Source: CAD feature listing. Evaluate the final solid. Frame: model axes, mm. A direction names the side the tool comes from. Round coordinates to 2 decimals unless told otherwise and drop trailing zeros. Write each loop counter-clockwise with the first axis right and the second up, starting at its lowest first coordinate (ties: lowest second). Pieces come first, ordered by that corner, then holes. Notation, with made-up numbers: M 81.5,79 L 87.5,79 A6 ccw 87.5,84 Z; hole C 69.25,19 d7. An arc over 180 degrees is marked long. Answer in a Markdown table with one row per item. Add a question column.
Item 1: Cut plane D-D on z = 0. Give the number of separate pieces and of enclosed holes in the cut face, and give its area (3 significant figures).
Item 2: Cut plane C-C on y = -10.75. Return loops of the section in (x, z), and give its area (3 significant figures).
Item 3: Cut plane B-B on z = 21.5. Return loops of the section in (x, y), and give its area (3 significant figures).
Item 4: Material intervals for probe 1 along X at (y, z) = (-14.45, 0); probe 2 along Y at (x, z) = (-3, -6.5); probe 3 along Z at (x, y) = (0, -0.9), sorted ascending.
Item 5: Contact query for flat-ended pins moving along their axis: pin 1 (2.5 mm diameter, centred on x = -30, z = 0, fed in from +Y); pin 2 (25 mm diameter, centred on x = -4, z = 11, fed in from +Y); pin 3 (1 mm diameter, centred on x = -28, y = -4, fed in from -Z). Output: stop coordinate, or through.
Item 6: Cut plane A-A on x = 30. Return loops of the section in (y, z).
Item 7: Mould query, pull axis Z, two halves, no side actions, for faces 3 (the face through (0, -1, -2)), 4 (the face through (-50, -14, 9)), 5 (the face through (-35, -7, 28.5)). Classes: released by +Z, released by -Z, zero draft, split by the parting line, or undercut.
Item 8: Set-up query: faces 1 (the face through (-1, 0, 5)), 2 (the face through (42, -7, 28.5)). Return all of +Z, -Z, +X, -X, +Y, -Y with unobstructed straight access to the full face (end or side cutting, diameter ignored); none if empty.
from build123d import *

# Parameters (mm, degrees)
F0_W     = 100
F0_H     = 50
F0_R     = 2
F0_R_2   = 2.212138
F1_DEPTH = 15
F2_W     = 12
F2_H     = 48.5
F3_DEPTH = 100.001
F4_W     = 55
F4_H     = 12
F5_DEPTH = 25


with BuildPart() as f1:
    # F0 (on Front) → F1 (new body)
    with BuildSketch(Plane.XZ):
        with Locations((0, 5)):
            Rectangle(F0_W, F0_H)
        with Locations((-30, 0)):
            Circle(F0_R, mode=Mode.SUBTRACT)
        Circle(F0_R, mode=Mode.SUBTRACT)
        with Locations((30, 0)):
            Circle(F0_R, mode=Mode.SUBTRACT)
        with Locations((20, 25)):
            Circle(F0_R_2, mode=Mode.SUBTRACT)
    extrude(amount=F1_DEPTH)

    # F2 (on face) → F3 (cut, through all)
    with BuildSketch(Plane(origin=(-50, 0, 0), x_dir=(0, -1, 0), z_dir=(-1, 0, 0))):
        with Locations((7.5, 4.25)):
            Rectangle(F2_W, F2_H)
    extrude(amount=-F3_DEPTH, mode=Mode.SUBTRACT)

    # F4 (on face) → F5 (cut)
    with BuildSketch(Plane.XY.offset(30)):
        with Locations((7.5, -7.5)):
            Rectangle(F4_W, F4_H)
    extrude(amount=-F5_DEPTH, mode=Mode.SUBTRACT)


solid = f1.part
Results below:
| question | item | result |
|---|---|---|
| 1 | separate pieces | 8 |
| 1 | enclosed holes | 0 |
| 1 | area | 264 mm2 |
| 2 | outline | M -50,28.5 L -20,28.5 L -20,30 L -50,30 Z; M 35,28.5 L 50,28.5 L 50,30 L 35,30 Z |
| 2 | area | 67.5 mm2 |
| 3 | outline | M -50,-15 L 50,-15 L 50,-13.5 L -50,-13.5 Z; M -50,-1.5 L 50,-1.5 L 50,0 L -50,0 Z |
| 3 | area | 300 mm2 |
| 4 | probe 1 | -50 to -32, -28 to -2, 2 to 28, 32 to 50 |
| 4 | probe 2 | -15 to -13.5, -1.5 to 0 |
| 4 | probe 3 | -20 to -2, 2 to 30 |
| 5 | pin 1 | through |
| 5 | pin 2 | y = 0 |
| 5 | pin 3 | z = 28.5 |
| 6 | outline | M -15,-20 L -13.5,-20 L -13.5,-2 L -15,-2 Z; M -15,2 L -13.5,2 L -13.5,30 L -15,30 Z; M -1.5,-20 L 0,-20 L 0,-2 L -1.5,-2 Z; M -1.5,2 L 0,2 L 0,30 L -1.5,30 Z |
| 7 | face 3 | undercut |
| 7 | face 4 | zero draft |
| 7 | face 5 | released by -Z |
| 8 | face 1 | +Z, -Z, +X, -X, +Y |
| 8 | face 2 | -Z, +X, -X |
